Read the model definition and answer for the solid it produces. Units are mm, in the model's axes. Face numbers are marked on the shaded views. A direction names the side the tool comes from. Round coordinates to 2 decimals unless told otherwise and drop trailing zeros. Write each loop counter-clockwise with the first axis right and the second up, starting at its lowest first coordinate (ties: lowest second). Pieces come first, ordered by that corner, then holes.
from build123d import *

# Parameters (mm, degrees)
SKETCH2_W           = 50.8
SKETCH2_H           = 101.6
BOSS_EXTRUDE1_DEPTH = 6.35
SKETCH4_W           = 38.1
SKETCH4_H           = 21.59
BOSS_EXTRUDE2_DEPTH = 50.8
SKETCH5_R           = 4
CUT_EXTRUDE1_DEPTH  = 88.779419712
SKETCH6_W           = 28.448
SKETCH6_H           = 15.71752
CUT_EXTRUDE2_DEPTH  = 77.2


with BuildPart() as part:
    # Sketch2 → Boss-Extrude1 (new body)
    with BuildSketch(Plane(origin=(0, 0, 0), x_dir=(1, 0, 0), z_dir=(0, 1, 0))):
        Rectangle(SKETCH2_W, SKETCH2_H)
    extrude(amount=BOSS_EXTRUDE1_DEPTH)

    # Sketch4 → Boss-Extrude2 (add)
    with BuildSketch(Plane(origin=(0, 6.35, 0), x_dir=(1, 0, 0), z_dir=(0, 1, 0))):
        with Locations((-6.35, 0)):
            Rectangle(SKETCH4_W, SKETCH4_H)
    extrude(amount=BOSS_EXTRUDE2_DEPTH)

    # Sketch5 → Cut-Extrude1 (cut, through all)
    with BuildSketch(Plane(origin=(0, 0, -10.795), x_dir=(-1, 0, 0), z_dir=(0, 0, -1))):
        with Locations((6.35, 31.75)):
            Circle(SKETCH5_R)
    extrude(amount=-CUT_EXTRUDE1_DEPTH, mode=Mode.SUBTRACT)

    # Sketch6 → Cut-Extrude2 (cut, through all)
    with BuildSketch(Plane(origin=(0, 6.35, 0), x_dir=(1, 0, 0), z_dir=(0, 1, 0))):
        with Locations((-6.35, 21.52396)):
            Rectangle(SKETCH6_W, SKETCH6_H)
    extrude(amount=-CUT_EXTRUDE2_DEPTH, mode=Mode.SUBTRACT)


solid = part.part
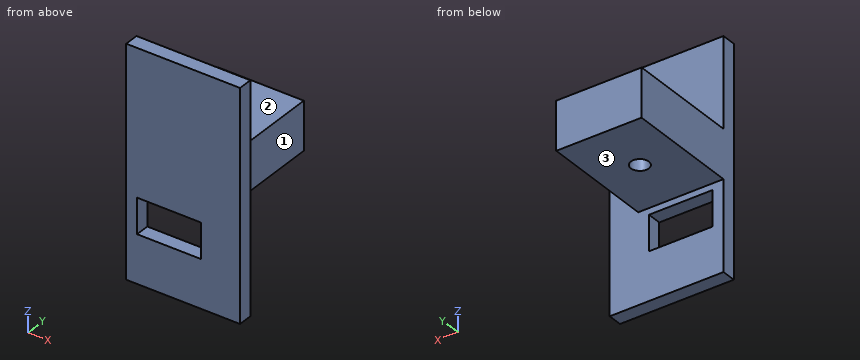
Q1. Section D-D (x = -6.35) is taken. Determine the outline of the cut face in (y, z) (3 decimals), then the cut area to 3 significant figures.
Verdict:
outline: (0, -50.8) - (6.35, -50.8) - (6.35, -29.383) - (0, -29.383) - close; (0, -13.665) - (6.35, -13.665) - (6.35, -10.795) - (27.75, -10.795) - (27.75, 10.795) - (6.35, 10.795) - (6.35, 50.8) - (0, 50.8) - close; (35.75, -10.795) - (57.15, -10.795) - (57.15, 10.795) - (35.75, 10.795) - close
area: 1,470 mm2
Q2. Flat-ended cylindrical pins translate along their axes: pin 1 Ø7 at (x, y) = (-6.35, 31.75) entering from -Z; pin 2 Ø1 at (x, y) = (7, 22.5) entering from -Z (3 decimals); pin 3 Ø1.5 at (x, y) = (1.5, 40.5) entering from +Z (3 decimals); pin 4 Ø8 at (y, z) = (44.5, -2.5) entering from +X. Find the tip coordinate at first contact, or state that the pin passes through.
Verdict:
pin 1: passes through
pin 2: stops at z = -10.795
pin 3: stops at z = 10.795
pin 4: stops at x = 12.7
Q3. Straight lines are drawn through the part: probe 1 along Y at (x, z) = (-6.35, 2.5); probe 2 along Z at (x, y) = (3.5, 3); probe 3 along X at (y, z) = (43.5, 8.5). For each, find the intervals that lie inside material, in ascending order.
Verdict:
probe 1: y = 0 to 27.75, 35.75 to 57.15
probe 2: z = -50.8 to -29.38, -13.67 to 50.8
probe 3: x = -25.4 to 12.7
Q4. Section A-A (x = 3) is taken. Determine the outline of the cut face in (y, z) (3 decimals).
Verdict:
outline: (0, -50.8) - (6.35, -50.8) - (6.35, -29.383) - (0, -29.383) - close; (0, -13.665) - (6.35, -13.665) - (6.35, -10.795) - (57.15, -10.795) - (57.15, 10.795) - (6.35, 10.795) - (6.35, 50.8) - (0, 50.8) - close
Q5. Section B-B (y = 31.75) is taken. Determine the outline of the cut face in (x, z) (3 decimals), then the cut area to 3 significant figures.
Verdict:
outline: (-25.4, -10.795) - (-10.35, -10.795) - (-10.35, 10.795) - (-25.4, 10.795) - close; (-2.35, -10.795) - (12.7, -10.795) - (12.7, 10.795) - (-2.35, 10.795) - close
area: 650 mm2
Q6. Which of the six approach directions +Z, -Z, +X, -X, +Y, -Y give full straight-line access (tool end or side, diameter ignored) to the marked faces 1, 2 and 3?
Verdict:
face 1: +Z, -Z, +X, +Y
face 2: +Z, +X, -X, +Y
face 3: -Z, +X, -X, +Y
Q7. Section C-C (z = 6) is taken. Determine the outline of the cut face in (x, y), then the cut area to 3 significant figures.
Verdict:
outline: (-25.4, 0) - (25.4, 0) - (25.4, 6.35) - (12.7, 6.35) - (12.7, 57.15) - (-25.4, 57.15) - close; hole circle Ø8 at (-6.35, 31.75)
area: 2,210 mm2
